Drawing for the job (mm, zero at the part's lowest x, y, z). A direction names the side the tool comes from. Coordinates: 2 decimals unless noted, no trailing zeros. Write each loop counter-clockwise with the first axis right and the second up, starting at its lowest first coordinate (ties: lowest second). Pieces come first, ordered by that corner, then holes. Notation, with made-up numbers: M 42,81.5 L 67,81.5 A27 ccw 67,97.5 Z; hole C 66.25,13.5 d6. An arc over 180 degrees is marked long. Use CSV: the item, a comma, the result in double quotes. Start each with the question number.
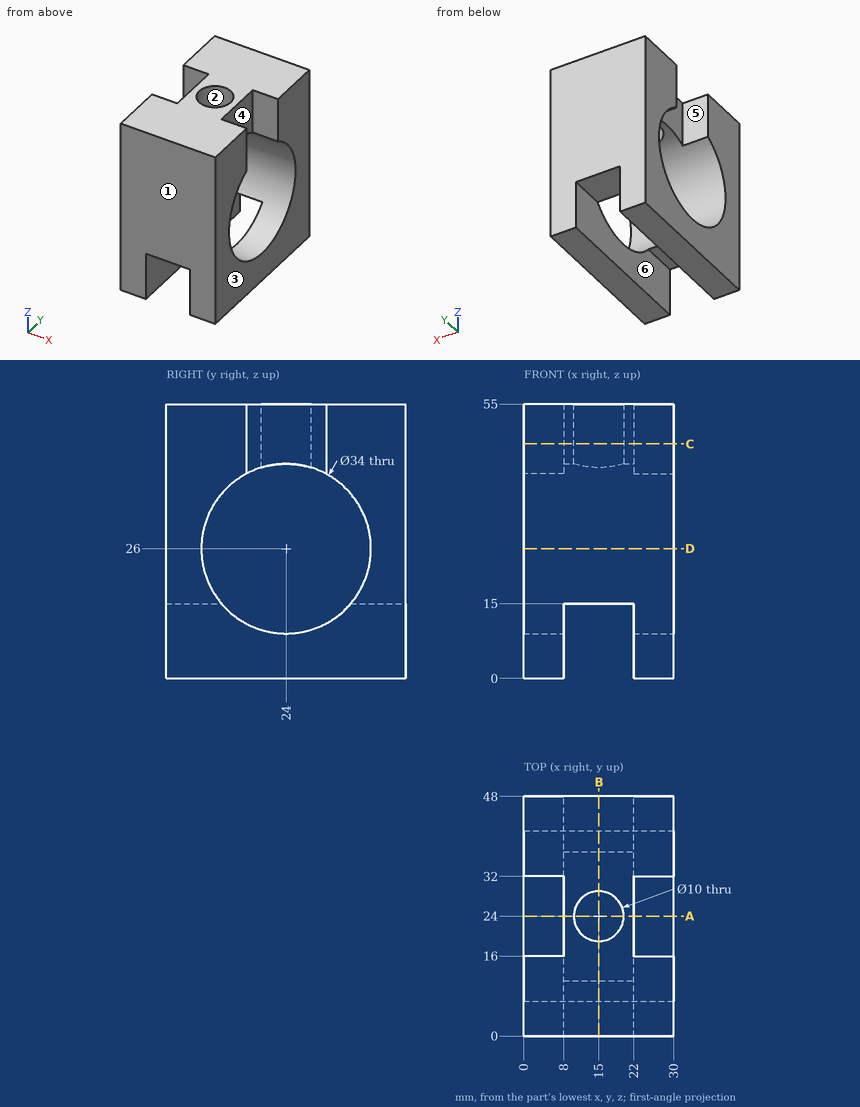
1) Band-saw the part on B-B on x = 15. List the corners of the cut face in (y, z).
2) Band-saw the part on A-A on y = 24. List the corners of the cut face in (x, z), then the cut area to 3 significant figures.
3) Tool access for the marked faces 4, 5 and 6: list every direction of +Z, -Z, +X, -X, +Y, -Y with a clear straight run to the whole face (end or side of a thin tool).
4) Wall check: L1, parallel to Y at x = 24, z = 11; L2, parallel to X at y = 9, z = 12.5; L3, parallel to Y at x = 7, z = 26. Give the ranges that are in metal, low to high. Write a range as [from, to].
5) Two-plate mould, pull along X, no slides. Class the marked faces 1, 2 and 3: pulls with the +X half, pulls with the -X half, needs draft (parallel to the pull), parting line crosses it, or undercut.
6) Drop flat-ended pins along their axis: P1, Ø3.5, axis at x = 15, y = 41.5, coming from the -Z side; P2, Ø1.5, axis at x = 19.5, y = 31.5, coming from the -Z side; P3, Ø7, axis at y = 24, z = 47.5, coming from the +X side. Give the stop position or say it passes through.
7) Band-saw the part on C-C on z = 47. List the corners of the cut face in (x, y).
8) Band-saw the part on D-D on z = 26. List the corners of the cut face in (x, y), then the cut area to 3 significant figures.
Findings below:
1,outline,"M 0,15 L 11.04,15 A17 cw 19,42.25 L 19,55 L 0,55 Z; M 29,42.25 A17 cw 36.96,15 L 48,15 L 48,55 L 29,55 Z"
2,outline,"M 0,0 L 8,0 L 8,9 L 0,9 Z; M 8,43 L 10,43 L 10,55 L 8,55 Z; M 20,43 L 22,43 L 22,55 L 20,55 Z; M 22,0 L 30,0 L 30,9 L 22,9 Z"
2,area,"192 mm2"
3,face 4,"+Z, +X"
3,face 5,"+Z, -X"
3,face 6,"-Z, +Y, -Y"
4,L1,"y = [0, 16], [32, 48]"
4,L2,"x = [0, 8], [22, 30]"
4,L3,"y = [0, 7], [41, 48]"
5,face 1,"needs draft"
5,face 2,"undercut"
5,face 3,"pulls with the +X half"
6,P1,"stops at z = 15"
6,P2,"stops at z = 40.86"
6,P3,"stops at x = 22"
7,outline,"M 0,0 L 30,0 L 30,16 L 22,16 L 22,32 L 30,32 L 30,48 L 0,48 L 0,32 L 8,32 L 8,16 L 0,16 Z; hole C 15,24 d10"
8,outline,"M 0,0 L 30,0 L 30,7 L 0,7 Z; M 0,41 L 30,41 L 30,48 L 0,48 Z"
8,area,"420 mm2"
